```python
from build123d import *

# Parameters (mm, degrees)
CROQUIS1_R                   = 50
SALIENTE_EXTRUIR1_DEPTH      = 30
SALIENTE_EXTRUIR2_REACH      = 144.478
SALIENTE_EXTRUIR2_END_RADIUS = 50
CROQUIS3_W                   = 60
CROQUIS3_H                   = 60
CROQUIS3_W_2                 = 50.8
CROQUIS3_H_2                 = 50.8
CROQUIS4_R                   = 45
CROQUIS4_R_2                 = 32.5
CORTAR_EXTRUIR1_DEPTH        = 1.5


with BuildPart() as part:
    # Croquis1 → Saliente-Extruir1 (new, symmetric)
    with BuildSketch(Plane(origin=(0, 0, 0), x_dir=(0, 0, -1), z_dir=(1, 0, 0))):
        Circle(CROQUIS1_R)
    extrude(amount=SALIENTE_EXTRUIR1_DEPTH, both=True)

    # Saliente-Extruir2: up to this cylinder (the profile starts outside it)
    saliente_extruir2_end = Plane(origin=(0, 0, 0), z_dir=(-1, 0, 0)) * Cylinder(SALIENTE_EXTRUIR2_END_RADIUS, 389.956, mode=Mode.PRIVATE)
    # Croquis3 → Saliente-Extruir2 (add, up to the surface)
    with BuildSketch(Plane(origin=(0, 80, 0), x_dir=(1, 0, 0), z_dir=(0, 1, 0)), mode=Mode.PRIVATE) as saliente_extruir2_sk1:
        Rectangle(CROQUIS3_W, CROQUIS3_H)
        Rectangle(CROQUIS3_W_2, CROQUIS3_H_2, mode=Mode.SUBTRACT)
    saliente_extruir2_tool1 = extrude(saliente_extruir2_sk1.sketch, amount=-SALIENTE_EXTRUIR2_REACH, mode=Mode.PRIVATE) - saliente_extruir2_end
    add(saliente_extruir2_tool1.solids().sort_by_distance((0, 80, 29.151472))[0])

    # Croquis4 → Cortar-Extruir1 (cut)
    with BuildSketch(Plane(origin=(30, 0, 0), x_dir=(0, 0, -1), z_dir=(1, 0, 0))):
        Circle(CROQUIS4_R)
        Circle(CROQUIS4_R_2, mode=Mode.SUBTRACT)
    extrude(amount=-CORTAR_EXTRUIR1_DEPTH, mode=Mode.SUBTRACT)


solid = part.part
```
The model under review builds one solid part; all positions refer to its coordinate system, in mm. A direction names the side the tool comes from. Round coordinates to 2 decimals unless told otherwise and drop trailing zeros. Write each loop counter-clockwise with the first axis right and the second up, starting at its lowest first coordinate (ties: lowest second). Pieces come first, ordered by that corner, then holes. Notation, with made-up numbers: (19.5, -13) - (25.5, -13) arc R18 ccw to (25.5, -9) - close; hole circle Ø7 at (25, 52.25). An arc over 180 degrees is marked (long way). One line per question, with ' | ' between items.
Item 1: For P1, Ø2, axis at x = 0, y = 46, coming from the +Z side; P2, Ø18.5, axis at x = 9.5, y = 62.5, coming from the -Z side; P3, Ø1.5, axis at x = -12, z = 2, coming from the +Y side, all flat-tipped, find the tip position at first contact; note any pin that passes through.
Resolved:
P1: stops at z = 30 | P2: stops at z = -30 | P3: stops at y = 49.98
Item 2: To check wall thickness, follow probe 1 along Y at (x, z) = (29.4, 0); probe 2 along Z at (x, y) = (7, 66.5); probe 3 along X at (y, z) = (24.5, -21.5). State the ranges of each line that lie inside material, in increasing order.
Resolved:
probe 1: y = -50 to -45, -32.5 to 32.5, 45 to 80 | probe 2: z = -30 to -25.4, 25.4 to 30 | probe 3: x = -30 to 28.5
Item 3: The part is to be moulded in two halves that separate along Y. For faces 5 (the face through (28.5, -30, -13)), 6 (the face through (-27, 80, 0)), 7 (the face through (29.26, -39.923, -20.765)), 8 (the face through (25.4, 66, 0)), say which applies: pulls with the +Y half, pulls with the -Y half, needs draft (parallel to the pull), parting line crosses it, or undercut.
Resolved:
face 5: undercut | face 6: pulls with the +Y half | face 7: undercut | face 8: needs draft
Item 4: Add section D-D, the plane y = -24.5. Give the boundary of the cut face in (x, z).
Resolved:
outline: (-30, -43.59) - (30, -43.59) - (30, -37.75) - (28.5, -37.75) - (28.5, -21.35) - (30, -21.35) - (30, 21.35) - (28.5, 21.35) - (28.5, 37.75) - (30, 37.75) - (30, 43.59) - (-30, 43.59) - close
Item 5: Add section C-C, the plane x = 14. Give the boundary of the cut face in (y, z).
Resolved:
outline: (40, -30) - (80, -30) - (80, -25.4) - (43.07, -25.4) arc R50 ccw to (43.07, 25.4) - (80, 25.4) - (80, 30) - (40, 30) arc R50 ccw (long way) to start
Item 6: For faces 1 (the face through (29.26, 9.76, -31)), 2 (the face through (0, 60, -30)), 3 (the face through (-25.4, 66, 0)), 4 (the face through (0, 60, 30)), list the 3-axis set-ups (+Z, -Z, +X, -X, +Y, -Y) from which the entire face can be reached by the end or side of a thin tool; tool diameter is ignored.
Resolved:
face 1: +X | face 2: -Z, +X, -X, +Y | face 3: +Y | face 4: +Z, +X, -X, +Y
Item 7: Add section A-A, the plane y = 56.5. Give the boundary of the cut face in (x, z), then the cut area to 3 significant figures.
Resolved:
outline: (-30, -30) - (30, -30) - (30, 30) - (-30, 30) - close; hole (-25.4, -25.4) - (25.4, -25.4) - (25.4, 25.4) - (-25.4, 25.4) - close | area: 1,020 mm2
Item 8: Add section B-B, the plane z = 0. Give the boundary of the cut face in (x, y).
Resolved:
outline: (-30, -50) - (30, -50) - (30, -45) - (28.5, -45) - (28.5, -32.5) - (30, -32.5) - (30, 32.5) - (28.5, 32.5) - (28.5, 45) - (30, 45) - (30, 80) - (25.4, 80) - (25.4, 50) - (-25.4, 50) - (-25.4, 80) - (-30, 80) - close
